Source: three-view drawing plus pictorial views. Frame: mm from the lowest corner of the part. A direction names the side the tool comes from. Round coordinates to 2 decimals unless told otherwise and drop trailing zeros. Write each loop counter-clockwise with the first axis right and the second up, starting at its lowest first coordinate (ties: lowest second). Pieces come first, ordered by that corner, then holes. Notation, with made-up numbers: (18, -22.5) -> (50, -22.5) arc R28 cw to (50, 15.5) -> close; hole circle Ø5 at (-27.5, 13.5). An arc over 180 degrees is marked (long way). Put each result on its own line as item: value.
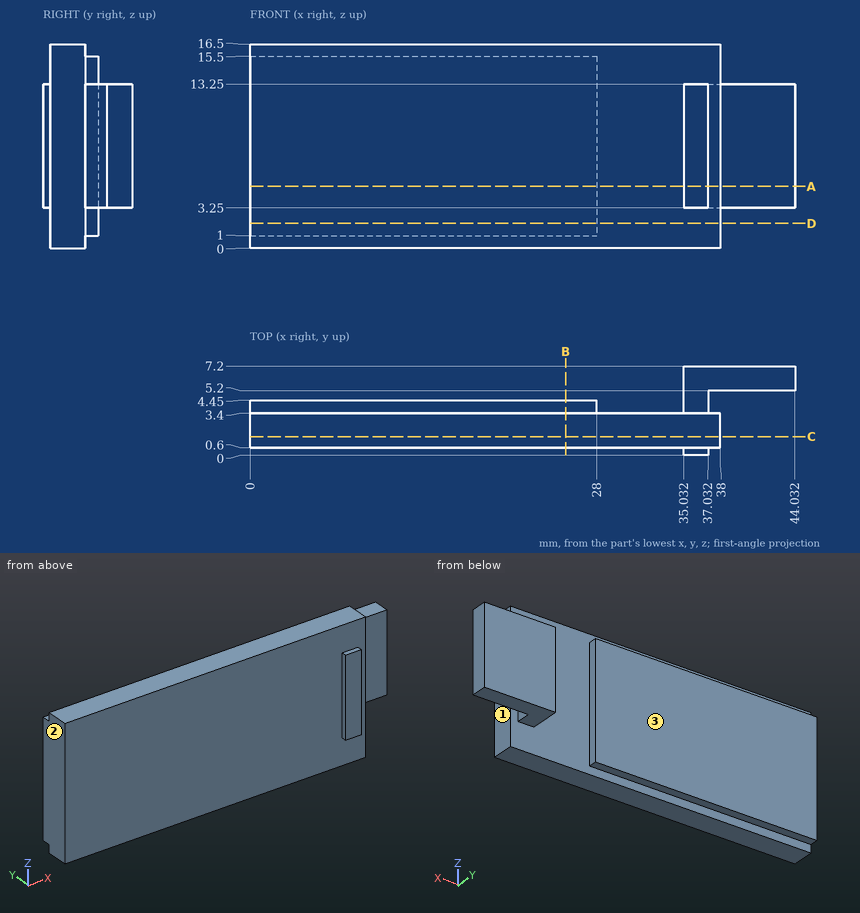
Q1. Reachability of the marked faces 1, 2 and 3 from +Z, -Z, +X, -X, +Y, -Y: full face, straight path, thin tool, end or side. Return the list, or none.
Ans:
face 1: +Z, -Z, +X, -Y
face 2: +Z, -Z, -X, +Y, -Y
face 3: +Z, -Z, -X, +Y
Q2. Pin query (flat end, axial travel): pin 1 (5.5 mm diameter, centred on x = 42, z = 10, fed in from -Y); pin 2 (1 mm diameter, centred on y = 2.5, z = 6.5, fed in from +X); pin 3 (8 mm diameter, centred on x = 7.5, z = 2, fed in from -Y). Return the tip coordinate at first contact, or that it passes through.
Ans:
pin 1: stops at y = 5.2
pin 2: stops at x = 38
pin 3: stops at y = 0.6
Q3. Cut plane B-B on x = 25.5. Output: boundary loops of the cut face in (y, z), and give its area (3 significant figures).
Ans:
outline: (0.6, 0) -> (3.4, 0) -> (3.4, 1) -> (4.45, 1) -> (4.45, 15.5) -> (3.4, 15.5) -> (3.4, 16.5) -> (0.6, 16.5) -> close
area: 61.4 mm^2
Q4. Material intervals for line 1 (X direction, y = 3.5, z = 9.25); line 2 (Y direction, x = 2, z = 14.5); line 3 (Y direction, x = 42, z = 4.25), sorted ascending. Write a range as [from, to].
Ans:
line 1: x = [0, 28], [35.03, 37.03]
line 2: y = [0.6, 4.45]
line 3: y = [5.2, 7.2]
Q5. Cut plane C-C on y = 1.5. Output: boundary loops of the cut face in (x, z), and give its area (3 significant figures).
Ans:
outline: (0, 0) -> (38, 0) -> (38, 16.5) -> (0, 16.5) -> close
area: 627 mm^2
Q6. Cut plane D-D on z = 2. Output: boundary loops of the cut face in (x, y), and give its area (3 significant figures).
Ans:
outline: (0, 0.6) -> (38, 0.6) -> (38, 3.4) -> (28, 3.4) -> (28, 4.45) -> (0, 4.45) -> close
area: 136 mm^2
Q7. Cut plane A-A on z = 5. Output: boundary loops of the cut face in (x, y).
Ans:
outline: (0, 0.6) -> (35.03, 0.6) -> (35.03, 0) -> (37.03, 0) -> (37.03, 0.6) -> (38, 0.6) -> (38, 3.4) -> (37.03, 3.4) -> (37.03, 5.2) -> (44.03, 5.2) -> (44.03, 7.2) -> (35.03, 7.2) -> (35.03, 3.4) -> (28, 3.4) -> (28, 4.45) -> (0, 4.45) -> close
